```python
from build123d import *

# Parameters (mm, degrees)
SM_START                     = -142
SM_BASE_FLANGE_1_DEPTH       = 284
SKETCH_6_R                   = 27
CUT_EXTRUDE_1_DEPTH          = 10
HOLE_WIZARD_5_5_5_5_1_D      = 5.5
HOLE_WIZARD_5_5_5_5_1_DEPTH  = 14
HOLE_WIZARD_5_5_5_5_1_TIP    = 1.652366702
HOLE_WIZARD_7_0_7_1_D        = 7
SKETCH_21_W                  = 210
SKETCH_21_H                  = 11
CUT_EXTRUDE_4_DEPTH          = 213.395480178
FILLET_1_R                   = 10
HOLE_WIZARD_M31_D            = 2.5
HOLE_WIZARD_M31_DEPTH        = 8.5
HOLE_WIZARD_M31_TIP          = 0.751075774
SM_EDGE_FLANGE_1_DEPTH       = 284
FILLET_3_R                   = 5
EXTRUDE_1_DEPTH              = 2
CUT_EXTRUDE_5_DEPTH          = 10
HOLE_WIZARD_6_1_6_1_1_D      = 6.1
HOLE_WIZARD_6_1_6_1_1_DEPTH  = 7.25
HOLE_WIZARD_6_1_6_1_1_TIP    = 1.832624888
F_10_5_10_5_DIAMETER_HOLE1_D = 10.5


# Read off the part's stored shape, not the designer's step: Базовая кромка1
# Sheet-metal steps are written as plain solids
with BuildPart() as part:
    # Базовая кромка1 outline → Базовая кромка1 (new body)
    with BuildSketch(Plane(origin=(0, 0, 0), x_dir=(0, 0, -1), z_dir=(1, 0, 0)).offset(SM_START)):
        with BuildLine():
            Line((4.4, 0), (40, 0))
            Line((40, 0), (40, 2))
            Line((40, 2), (4.4, 2))
            ThreePointArc((4.4, 2), (2.702943725, 2.702943725), (2, 4.4))
            Line((2, 4.4), (2, 152.8))
            Line((2, 152.8), (0, 152.8))
            Line((0, 152.8), (0, 4.4))
            ThreePointArc((0, 4.4), (1.288730163, 1.288730163), (4.4, 0))
        make_face()
    extrude(amount=SM_BASE_FLANGE_1_DEPTH)

    # Эскиз6 → Вырез-Вытянуть1 (cut)
    with BuildSketch(Plane.XY):
        with Locations((0, 44)):
            Circle(SKETCH_6_R)
    extrude(amount=-CUT_EXTRUDE_1_DEPTH, mode=Mode.SUBTRACT)

    # Диаметр отверстия Ø5.5 (5.5)1
    with Locations(Plane.XY):
        with Locations((131.35, 91), (-131.35, 91), (-131.35, 26), (131.35, 26)):
            Hole(HOLE_WIZARD_5_5_5_5_1_D / 2, depth=HOLE_WIZARD_5_5_5_5_1_DEPTH)
            with Locations((0, 0, -(HOLE_WIZARD_5_5_5_5_1_DEPTH + HOLE_WIZARD_5_5_5_5_1_TIP / 2))):  # 118° drill point
                Cone(0, HOLE_WIZARD_5_5_5_5_1_D / 2, HOLE_WIZARD_5_5_5_5_1_TIP, mode=Mode.SUBTRACT)

    # Диаметр отверстия Ø7.0 (7)1 (through all)
    with Locations(Plane(origin=(0, 0, 0), x_dir=(-1, 0, 0), z_dir=(0, -1, 0))):
        with Locations((126, 28), (126, 13), (-126, 13), (-126, 28)):
            Hole(HOLE_WIZARD_7_0_7_1_D / 2)

    # Эскиз21 → Вырез-Вытянуть4 (cut, through all)
    with BuildSketch(Plane.XY):
        with Locations((0, 5.5)):
            Rectangle(SKETCH_21_W, SKETCH_21_H)
    extrude(amount=-CUT_EXTRUDE_4_DEPTH, mode=Mode.SUBTRACT)

    # Скругление1
    fillet_1_edges = [part.edges().sort_by_distance(p)[0] for p in [
        (-105, 1, -40),
        (105, 1, -40),
        (142, 1, -40),
        (-142, 1, -40),
    ]]
    fillet(fillet_1_edges, radius=FILLET_1_R)

    # Отверстие обработанное метчиком M31
    with Locations(Plane.XY):
        with Locations((-11.5, 85), (11.5, 85)):
            Hole(HOLE_WIZARD_M31_D / 2, depth=HOLE_WIZARD_M31_DEPTH)
            with Locations((0, 0, -(HOLE_WIZARD_M31_DEPTH + HOLE_WIZARD_M31_TIP / 2))):  # 118° drill point
                Cone(0, HOLE_WIZARD_M31_D / 2, HOLE_WIZARD_M31_TIP, mode=Mode.SUBTRACT)

    # Ребро-кромка1 section (across the edge) → Ребро-кромка1 (add)
    with BuildSketch(Plane(origin=(142, 155.2, 0), x_dir=(0, -1, 0), z_dir=(-1, 0, 0))):
        with BuildLine():
            Line((-2, 2.4), (-2, 23))
            Line((-2, 23), (0, 23))
            Line((0, 23), (0, 2.4))
            ThreePointArc((0, 2.4), (0.702943725, 0.702943725), (2.4, 0))
            Line((2.4, 0), (2.4, -2))
            ThreePointArc((2.4, -2), (-0.711269837, -0.711269837), (-2, 2.4))
        make_face()
    extrude(amount=SM_EDGE_FLANGE_1_DEPTH)

    # Скругление3
    fillet_3_edges = [part.edges().sort_by_distance(p)[0] for p in [
        (142, 156.2, 23),
        (-142, 156.2, 23),
    ]]
    fillet(fillet_3_edges, radius=FILLET_3_R)

    # Эскиз27 → Бобышка-Вытянуть1 (add)
    with BuildSketch(Plane.XY):
        with BuildLine():
            Line((40, 11), (-40, 11))
            ThreePointArc((-40, 11), (-34.734783955, 10.153684985), (-30, 7.7))
            ThreePointArc((-30, 7.7), (-25.265216045, 5.246315015), (-20, 4.4))
            Line((-20, 4.4), (20, 4.4))
            ThreePointArc((20, 4.4), (25.265216045, 5.246315015), (30, 7.7))
            ThreePointArc((30, 7.7), (34.734783955, 10.153684985), (40, 11))
        make_face()
    extrude(amount=-EXTRUDE_1_DEPTH)

    # Эскиз28 → Вырез-Вытянуть5 (cut)
    with BuildSketch(Plane.XY):
        with BuildLine():
            Line((-112, 134.8), (-112, 39.919592204))
            ThreePointArc((-112, 39.919592204), (-109.632057622, 36.986930757), (-106.266331225, 38.683851525))
            Line((-106.266331225, 38.683851525), (-63.376138879, 133.564259321))
            ThreePointArc((-63.376138879, 133.564259321), (-63.589170628, 136.426772566), (-66.109807654, 137.8))
            Line((-66.109807654, 137.8), (-109, 137.8))
            ThreePointArc((-109, 137.8), (-111.121320344, 136.921320344), (-112, 134.8))
        make_face()
        with BuildLine():
            Line((-90.890192346, 26), (-72.924698752, 26))
            ThreePointArc((-72.924698752, 26), (-71.054378606, 26.65438653), (-70, 28.332064967))
            Line((-70, 28.332064967), (-51.656189361, 108.654427819))
            ThreePointArc((-51.656189361, 108.654427819), (-53.624269894, 112.16575547), (-57.314556889, 110.558103531))
            Line((-57.314556889, 110.558103531), (-93.623861121, 30.235740679))
            ThreePointArc((-93.623861121, 30.235740679), (-93.410829372, 27.373227434), (-90.890192346, 26))
        make_face()
        with BuildLine():
            Line((-27, 137.8), (27, 137.8))
            ThreePointArc((27, 137.8), (29.121320344, 136.921320344), (30, 134.8))
            Line((30, 134.8), (30, 105.8))
            ThreePointArc((30, 105.8), (29.121320344, 103.678679656), (27, 102.8))
            Line((27, 102.8), (-27, 102.8))
            ThreePointArc((-27, 102.8), (-29.121320344, 103.678679656), (-30, 105.8))
            Line((-30, 105.8), (-30, 134.8))
            ThreePointArc((-30, 134.8), (-29.121320344, 136.921320344), (-27, 137.8))
        make_face()
        with BuildLine():
            Line((70, 28.332064967), (51.656189361, 108.654427819))
            ThreePointArc((51.656189361, 108.654427819), (53.624269894, 112.16575547), (57.314556889, 110.558103531))
            Line((57.314556889, 110.558103531), (93.623861121, 30.235740679))
            ThreePointArc((93.623861121, 30.235740679), (93.410829372, 27.373227434), (90.890192346, 26))
            Line((90.890192346, 26), (72.924698752, 26))
            ThreePointArc((72.924698752, 26), (71.054378606, 26.65438653), (70, 28.332064967))
        make_face()
        with BuildLine():
            Line((112, 134.8), (112, 39.919592204))
            ThreePointArc((112, 39.919592204), (109.632057622, 36.986930757), (106.266331225, 38.683851525))
            Line((106.266331225, 38.683851525), (63.376138879, 133.564259321))
            ThreePointArc((63.376138879, 133.564259321), (63.589170628, 136.426772566), (66.109807654, 137.8))
            Line((66.109807654, 137.8), (109, 137.8))
            ThreePointArc((109, 137.8), (111.121320344, 136.921320344), (112, 134.8))
        make_face()
    extrude(amount=-CUT_EXTRUDE_5_DEPTH, mode=Mode.SUBTRACT)

    # Диаметр отверстия Ø6.1 (6.1)1
    with Locations(Plane(origin=(0, 157.2, 0), x_dir=(1, 0, 0), z_dir=(0, 1, 0))):
        with Locations((-129, -13.5), (-43, -13.5), (43, -13.5), (129, -13.5)):
            Hole(HOLE_WIZARD_6_1_6_1_1_D / 2, depth=HOLE_WIZARD_6_1_6_1_1_DEPTH)
            with Locations((0, 0, -(HOLE_WIZARD_6_1_6_1_1_DEPTH + HOLE_WIZARD_6_1_6_1_1_TIP / 2))):  # 118° drill point
                Cone(0, HOLE_WIZARD_6_1_6_1_1_D / 2, HOLE_WIZARD_6_1_6_1_1_TIP, mode=Mode.SUBTRACT)

    # Ø10.5 (10.5) Diameter Hole1 (through all)
    with Locations(Plane.XY):
        with Locations((-49.5, 44), (49.5, 44)):
            Hole(F_10_5_10_5_DIAMETER_HOLE1_D / 2)


solid = part.part
```
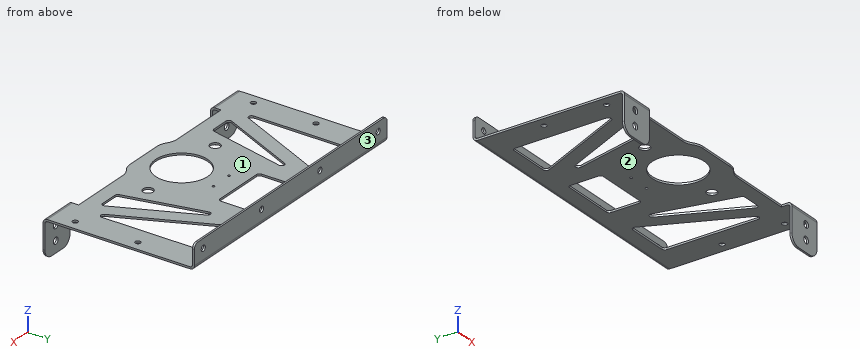
Here's how the part is built. I have some questions about the finished solid (model axes, mm). Face numbers are marked on the shaded views. A direction names the side the tool comes from. Round coordinates to 2 decimals unless told otherwise and drop trailing zeros. Order: outer loops, then holes, each group sorted by start corner. A loop starts at its lowest first (then second) coordinate and runs counter-clockwise, first axis right, second up. Notation, with made-up numbers: M 79,49 L 102,49 A4 cw 102,53 Z; hole C 21,62.5 d1. An arc over 180 degrees is marked long. Answer as CSV lines item,"result".
Item 1: Which directions (+Z, -Z, +X, -X, +Y, -Y) give clear straight access to the entire face, cutting with the end or side of a thin tool? Please do the marked faces 1, 2 and 3.
From the geometry:
face 1,"+Z, +X, -X, -Y"
face 2,"-Z, +X, -X, +Y"
face 3,"+Z, -Z, +X, -X, +Y"
Item 2: Imagine slicing it at B-B on x = 0. List the corners of the cut face in (y, z) for me.
From the geometry:
outline,"M 4.4,-2 L 17,-2 L 17,0 L 4.4,0 Z; M 71,-2 L 102.8,-2 L 102.8,0 L 71,0 Z; M 137.8,-2 L 152.8,-2 A4.4 ccw 157.2,2.4 L 157.2,23 L 155.2,23 L 155.2,2.4 A2.4 cw 152.8,0 L 137.8,0 Z"
Item 3: Imagine slicing it at C-C on y = 74.5. List the corners of the cut face in (x, z) for me, and give its area (3 significant figures).
From the geometry:
outline,"M -142,-2 L -112,-2 L -112,0 L -142,0 Z; M -90.08,-2 L -73.61,-2 L -73.61,0 L -90.08,0 Z; M -59.46,-2 L 59.46,-2 L 59.46,0 L -59.46,0 Z; M 73.61,-2 L 90.08,-2 L 90.08,0 L 73.61,0 Z; M 112,-2 L 142,-2 L 142,0 L 112,0 Z"
area,"424 mm2"
Item 4: Please list where these lines run through material, in increasing order: L1, parallel to Z at x = -43, y = 156.45; L2, parallel to Z at x = -114, y = 39.5; L3, parallel to Y at x = -52, z = 8.5. Write a range as [from, to].
From the geometry:
L1,"[-0.06, 10.45], [16.55, 23]"
L2,"[-2, 0]"
L3,"[155.2, 157.2]"
Item 5: Imagine slicing it at A-A on z = -13. List the corners of the cut face in (x, y) for me.
From the geometry:
outline,"M -142,0 L -129.5,0 L -129.5,2 L -142,2 Z; M -122.5,0 L -105,0 L -105,2 L -122.5,2 Z; M 105,0 L 122.5,0 L 122.5,2 L 105,2 Z; M 129.5,0 L 142,0 L 142,2 L 129.5,2 Z"
Item 6: For pin 1 (4.5 mm diameter, centred on x = 131.35, y = 26, fed in from -Z); pin 2 (12 mm diameter, centred on x = -37.5, y = 26.5, fed in from +Z); pin 3 (18 mm diameter, centred on x = -115, z = -28, fed in from +Y); pin 4 (1.5 mm diameter, centred on x = -40.5, y = 27.5, fed in from -Z), each with a flat end and sliding along its axis, tell me the tip position at first contact or that it passes through.
From the geometry:
pin 1,"through"
pin 2,"z = 0"
pin 3,"y = 2"
pin 4,"z = -2"
Item 7: Imagine slicing it at D-D on z = 13.5. List the corners of the cut face in (x, y) for me.
From the geometry:
outline,"M -142,155.2 L -132.05,155.2 L -132.05,157.2 L -142,157.2 Z; M -125.95,155.2 L -46.05,155.2 L -46.05,157.2 L -125.95,157.2 Z; M -39.95,155.2 L 39.95,155.2 L 39.95,157.2 L -39.95,157.2 Z; M 46.05,155.2 L 125.95,155.2 L 125.95,157.2 L 46.05,157.2 Z; M 132.05,155.2 L 142,155.2 L 142,157.2 L 132.05,157.2 Z"
